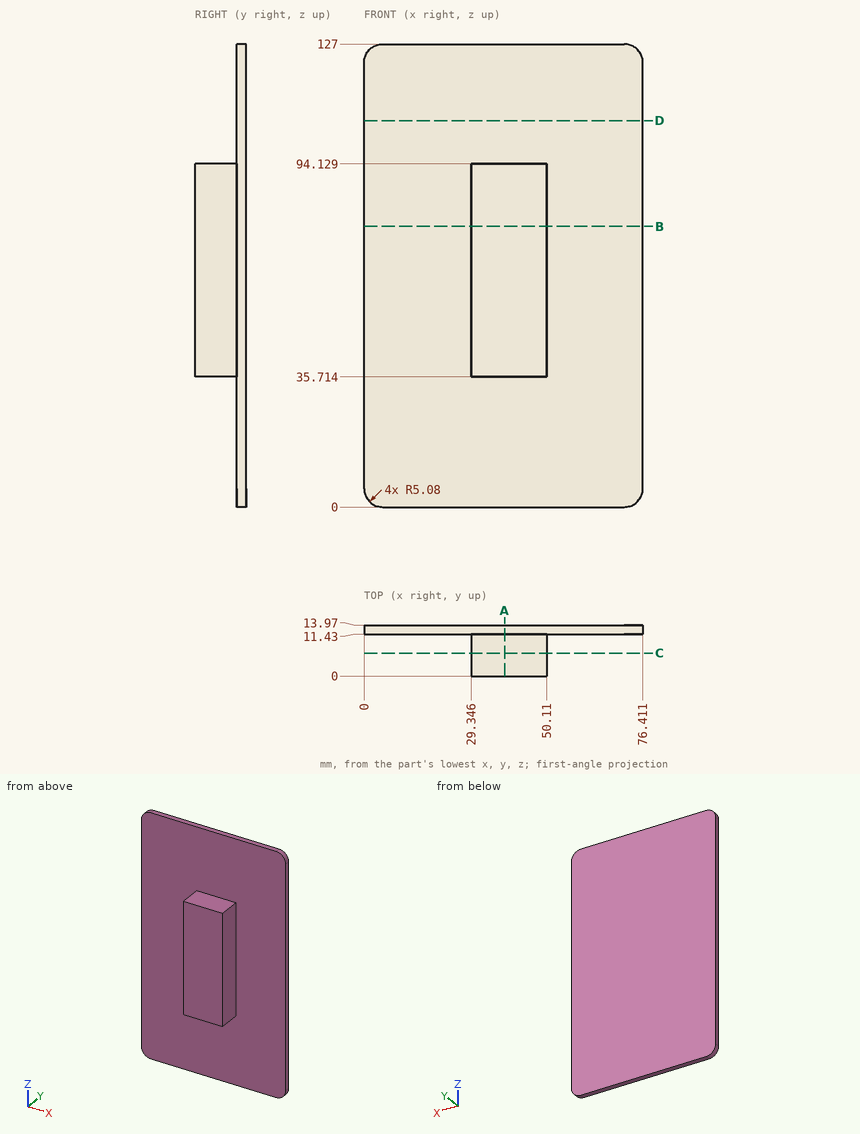
Geometry: see drawing. Coordinates: mm, zero at the bounding-box minimum. Round coordinates to 2 decimals unless told otherwise and drop trailing zeros. Loops run counter-clockwise (first coordinate to the right, second up) from the corner with the lowest first, then second, coordinate; pieces in that order, holes last.
(1) Material intervals for probe 1 along Y at (x, z) = (12.5, 39.5); probe 2 along X at (y, z) = (6.75, 56.5); probe 3 along Z at (x, y) = (30, 1.25), sorted ascending.
From the geometry:
probe 1: y = 11.43 to 13.97
probe 2: x = 29.35 to 50.11
probe 3: z = 35.71 to 94.13
(2) Section query C-C (y = 6.25). Output: boundary loops of the cut face in (x, z), and give its area (3 significant figures).
From the geometry:
outline: (29.35, 35.71) - (50.11, 35.71) - (50.11, 94.13) - (29.35, 94.13) - close
area: 1,210 mm2
(3) Section query B-B (z = 77). Output: boundary loops of the cut face in (x, y).
From the geometry:
outline: (0, 11.43) - (29.35, 11.43) - (29.35, 0) - (50.11, 0) - (50.11, 11.43) - (76.41, 11.43) - (76.41, 13.97) - (0, 13.97) - close
(4) Section query A-A (x = 38.5). Output: boundary loops of the cut face in (y, z).
From the geometry:
outline: (0, 35.71) - (11.43, 35.71) - (11.43, 0) - (13.97, 0) - (13.97, 127) - (11.43, 127) - (11.43, 94.13) - (0, 94.13) - close
(5) Contact query for flat-ended pins moving along their axis: pin 1 Ø3.5 at (x, y) = (38.5, 8) entering from -Z; pin 2 Ø5.5 at (x, y) = (38, 4.5) entering from +Z; pin 3 Ø4 at (y, z) = (3.5, 47.5) entering from -X. Output: stop coordinate, or through.
From the geometry:
pin 1: stops at z = 35.71
pin 2: stops at z = 94.13
pin 3: stops at x = 29.35
(6) Section query D-D (z = 106). Output: boundary loops of the cut face in (x, y).
From the geometry:
outline: (0, 11.43) - (76.41, 11.43) - (76.41, 13.97) - (0, 13.97) - close
